```python
from build123d import *

# Parameters (mm, degrees)
ESQUISSE2_W             = 5.5
ESQUISSE2_H             = 0.8
ENLEV_MAT_EXTRU_1_DEPTH = 1.3
ESQUISSE3_W             = 1.5
ESQUISSE3_H             = 10
CHANFREIN1_SIZE         = 0.3


with BuildPart() as part:
    # Esquisse1 → Base-R_volution (revolve)
    with BuildSketch(Plane(origin=(0, 0, 0), x_dir=(1, 0, 0), z_dir=(0, 1, 0)), mode=Mode.PRIVATE) as base_r_volution_sk:
        with BuildLine():
            Line((0, 0), (2.75, 0))
            Line((2.75, 0), (2.590995378, 1.817431149))
            ThreePointArc((2.590995378, 1.817431149), (2.52687448, 1.947455467), (2.391756438, 2))
            Line((2.391756438, 2), (0, 2))
            Line((0, 2), (0, 0))
        make_face()
    revolve(base_r_volution_sk.sketch.rotate(Axis((0, 0, 0), (0, 0, -1)), 180), axis=Axis((0, 0, 0), (0, 0, -1)))

    # Esquisse2 → Enlev. mat.-Extru.1 (cut)
    with BuildSketch(Plane.XY.offset(-2)):
        Rectangle(ESQUISSE2_W, ESQUISSE2_H)
    extrude(amount=ENLEV_MAT_EXTRU_1_DEPTH, mode=Mode.SUBTRACT)

    # Esquisse3 → Boss.-R_vol.1 (revolve)
    with BuildSketch(Plane(origin=(0, 0, 0), x_dir=(1, 0, 0), z_dir=(0, 1, 0)), mode=Mode.PRIVATE) as boss_r_vol_1_sk:
        with Locations((0.75, -5)):
            Rectangle(ESQUISSE3_W, ESQUISSE3_H)
    revolve(boss_r_vol_1_sk.sketch.rotate(Axis((0, 0, 0), (0, 0, 1)), 351.4444875), axis=Axis((0, 0, 0), (0, 0, 1)))

    # Chanfrein1
    chanfrein1_edges = [part.edges().sort_by_distance(p)[0] for p in [
        (-1.483308285, 0.223151363, 10),
    ]]
    chamfer(chanfrein1_edges, length=CHANFREIN1_SIZE)


solid = part.part
```
Could you check a few things on this model? Use its own coordinates, in mm. A direction names the side the tool comes from. Coordinates: 2 decimals unless noted, no trailing zeros. Loops run counter-clockwise (first coordinate to the right, second up) from the corner with the lowest first, then second, coordinate; pieces in that order, holes last. Notation, with made-up numbers: M 78,83.25 L 123,83.25 A22 ccw 123,117.25 Z; hole C -3,9 d4. An arc over 180 degrees is marked long. Put each result on its own line as item: value. Start each with the question number.
(1) Suppose I cut it at D-D on z = 2.5. Please give me the cut outline in (x, y).
(2) I need wall thicknesses on line 1 (Z direction, x = 2.25, y = 0.7); line 2 (Z direction, x = -1.95, y = 0.3); line 3 (Y direction, x = 0, z = 1). Which ranges of each line are inside material? Lowest first, please. Write a range as from..to.
(3) Suppose I cut it at A-A on x = 0. Please give me the cut outline in (y, z), then the cut area to 3 significant figures.
(4) Suppose I cut it at C-C on z = -0.25. Please give me the cut outline in (x, y), then the cut area to 3 significant figures.
(5) Will these pins go through, and if not, where does the flat tip stop? P1, Ø1.4, axis at x = -1, z = -1.5, coming from the -Y side; P2, Ø2, axis at y = 2, z = 5.5, coming from the +X side; P3, Ø0.7, axis at x = 0, z = -1.5, coming from the +Y side.
(6) Suppose I cut it at B-B on y = 0. Please give me the cut outline in (x, z).
(7) For faces 1 (the face through (0, 0.4, -1)), 2 (the face through (1.2, -1.2, 0)), 3 (the face through (0, -1, -2)), which set-ups out of +Z, -Z, +X, -X, +Y, -Y let a thin tool reach every point of the face, with its end or its side?
(8) Thinking about a two-plate mould opening in Y: for faces 4 (the face through (1.285, -0.774, 4.782)), 5 (the face through (0, 0, -0.7)), 6 (the face through (0, 1, -2)), 7 (the face through (0, -0.4, -1)), which applies, pulls with the +Y half, pulls with the -Y half, needs draft (parallel to the pull), parting line crosses it, or undercut?
Solutions:
1. outline: C 0,0 d3
2. line 1: z = -2..0
2. line 2: z = -0.7..0
2. line 3: y = -1.5..1.5
3. outline: M -2.75,0 L -2.59,-1.82 A0.2 ccw -2.39,-2 L -0.4,-2 L -0.4,-0.7 L 0.4,-0.7 L 0.4,-2 L 2.39,-2 A0.2 ccw 2.59,-1.82 L 2.75,0 L 1.5,0 L 1.5,9.7 L 1.2,10 L -1.2,10 L -1.5,9.7 L -1.5,0 Z
3. area: 39.5 mm2
4. outline: C 0,0 d5.46
4. area: 23.4 mm2
5. P1: stops at y = -2.62
5. P2: stops at x = 1.12
5. P3: stops at y = 2.65
6. outline: M -2.75,0 L -2.69,-0.7 L 2.69,-0.7 L 2.75,0 L 1.5,0 L 1.5,9.7 L 1.2,10 L -1.2,10 L -1.5,9.7 L -1.5,0 Z
7. face 1: -Z, +X, -X
7. face 2: +Z
7. face 3: -Z, +X, -X, +Y, -Y
8. face 4: parting line crosses it
8. face 5: undercut
8. face 6: needs draft
8. face 7: undercut
